Autodesk Fusion 360 part; units mm, degrees
sketch "Sketch1" plane through (0, 0, 0) normal (0, 0, 1) x (1, 0, 0)
  line L0 (-22.75, -6) -> (22.75, -6)
  arc A0 (22.75, -6) -> (22.75, 6) centre (22.75, 0) ccw
  line L1 (22.75, 6) -> (-22.75, 6)
  arc A1 (-22.75, 6) -> (-22.75, -6) centre (-22.75, 0) ccw
  line L2 (-22.75, 0) -> (22.75, 0) construction
  dimension "d1" = 45.5
  dimension "d2" = 12
extrude "Extrude1" add sketch "Sketch1" along normal blind 5
hole "Hole1" at (22.75, 0, 0) at (-22.75, 0, 0) direction (0, 0, 1) diameter 4.5 depth 8 tip angle 118
sketch "Sketch4" plane through (0, 0, 5) normal (0, 0, 1) x (-1, 0, 0)
  circle A0 centre (-22.75, 0) radius 2.25
  circle A1 centre (22.75, 0) radius 2.25
  arc A2 (22.75, -6) -> (22.75, 6) centre (22.75, 0) ccw
  line L0 (22.75, 6) -> (-22.75, 6)
  arc A3 (-22.75, 6) -> (-22.75, -6) centre (-22.75, 0) ccw
  line L1 (-22.75, -6) -> (22.75, -6)
  line L2 (-26.7048, 0) -> (-24.7274, -3.425)
  line L3 (-24.7274, -3.425) -> (-20.7726, -3.425)
  line L4 (-20.7726, -3.425) -> (-18.7952, 0)
  line L5 (-18.7952, 0) -> (-20.7726, 3.425)
  line L6 (-20.7726, 3.425) -> (-24.7274, 3.425)
  line L7 (-24.7274, 3.425) -> (-26.7048, 0)
  line L8 (-20.1952, 4.425) -> (-25.3048, 4.425)
  line L9 (-25.3048, 4.425) -> (-27.8595, 0)
  line L10 (-27.8595, 0) -> (-25.3048, -4.425)
  line L11 (-25.3048, -4.425) -> (-20.1952, -4.425)
  line L12 (-20.1952, -4.425) -> (-17.6405, 0)
  line L13 (-17.6405, 0) -> (-20.1952, 4.425)
  point P0 (-22.75, 0)
  dimension "d8" = 6.85
  dimension "d9" = 1
extrude "Extrude2" add sketch "Sketch4" along normal blind 4 contours L8 L9 L10 L11 L12 L13
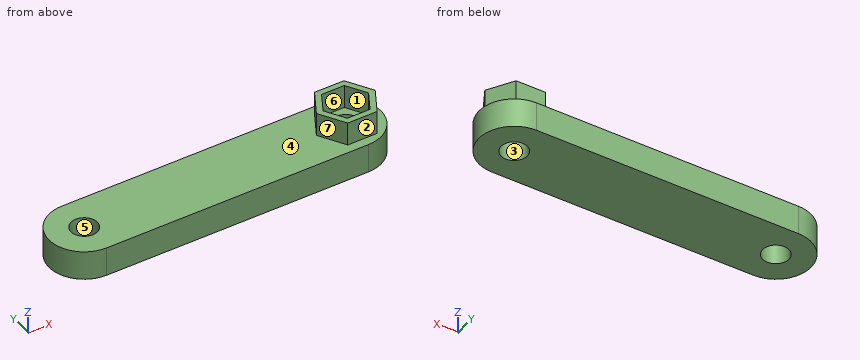
The model under review builds one solid part; all positions refer to its coordinate system, in mm. Face numbers are marked on the shaded views. A direction names the side the tool comes from. Give positions to 0.01 mm unless a question says otherwise; leave off trailing zeros. Order: outer loops, then holes, each group sorted by start corner. A loop starts at its lowest first (then second) coordinate and runs counter-clockwise, first axis right, second up. Notation, with made-up numbers: M 80.5,8 L 127.5,8 A20 cw 127.5,46 Z; hole C 85,-9.5 d4. An arc over 180 degrees is marked long. Use one line per item in the form item = value. Start each with the question number.
Item 1: We need section B-B on z = 4.5. Give the boundary of the cut face in (x, y), plus the area to 3 significant figures.
Item 2: Insertion check: pin 1 Ø3.5 at (x, y) = (24, -1) entering from +Z; pin 2 Ø4.5 at (x, z) = (23.5, 7.5) entering from +Y (3 decimals); pin 3 Ø3.5 at (x, y) = (22.75, 0) entering from -Z; pin 4 Ø1 at (y, z) = (1.5, 1.5) entering from +X. Each pin has a flat end and moves straight along its axis. Give the tip position at first contact, or say it passes through.
Item 3: We need section C-C on x = -21.5. Give the boundary of the cut face in (y, z).
Item 4: We need section D-D on x = -15. Give the boundary of the cut face in (y, z).
Item 5: For the marked faces 5, 6 and 7, list the 3-axis set-ups (+Z, -Z, +X, -X, +Y, -Y) from which the entire face can be reached by the end or side of a thin tool; tool diameter is ignored.
Item 6: The part is to be moulded in two halves that separate along Y. For the marked faces 1, 2, 3 and 4, say which applies: pulls with the +Y half, pulls with the -Y half, needs draft (parallel to the pull), parting line crosses it, or undercut.
Item 7: We need section A-A on y = 0.75. Give the boundary of the cut face in (x, z), plus the area to 3 significant figures.
Item 8: To check wall thickness, follow line 1 along X through (y, z) = (0, 1.5); line 2 along Y through (x, z) = (-22.75, 2.95); line 3 along Y through (x, z) = (21, 7.5) (3 decimals). State the ranges of each line that lie inside material, in increasing order. Write a range as from..to.
Completed:
q1.outline = M -22.75,-6 L 22.75,-6 A6 ccw 22.75,6 L -22.75,6 A6 ccw Z; hole C -22.75,0 d4.5; hole C 22.75,0 d4.5
q1.area = 627 mm²
q2.pin_1 = 5
q2.pin_2 = 4.425
q2.pin_3 = through
q2.pin_4 = 28.67
q3.outline = M -6,0 L -1.87,0 L -1.87,5 L -6,5 Z; M 1.87,0 L 6,0 L 6,5 L 1.87,5 Z
q4.outline = M -6,0 L 6,0 L 6,5 L -6,5 Z
q5.face_5 = +Z, -Z
q5.face_6 = +Z
q5.face_7 = +Z, -X, -Y
q6.face_1 = undercut
q6.face_2 = pulls with the -Y half
q6.face_3 = undercut
q6.face_4 = needs draft
q7.outline = M -28.7,0 L -24.87,0 L -24.87,5 L -28.7,5 Z; M -20.63,0 L 20.63,0 L 20.63,5 L 19.23,5 L 19.23,9 L 18.07,9 L 18.07,5 L -20.63,5 Z; M 24.87,0 L 28.7,0 L 28.7,5 L 27.43,5 L 27.43,9 L 26.27,9 L 26.27,5 L 24.87,5 Z
q7.area = 254 mm²
q8.line_1 = -28.75..-25, -20.5..20.5, 25..28.75
q8.line_2 = -6..-2.25, 2.25..6
q8.line_3 = -4.425..-3.425, 3.425..4.425
